Work out the finished part from the listing and answer in its coordinate system (mm). Round coordinates to 2 decimals unless told otherwise and drop trailing zeros. Order: outer loops, then holes, each group sorted by start corner. A loop starts at its lowest first (then second) coordinate and runs counter-clockwise, first axis right, second up. Notation, with made-up numbers: (-34.75, -4) - (-13.75, -4) arc R35 cw to (-13.75, 29) - close; hole circle Ø5 at (51, 85.5). An arc over 180 degrees is marked (long way). Use CSV: the item, a comma, the result in double quotes.
from build123d import *

# Parameters (mm, degrees)
CYLINDER107_R          = 1.8
CYLINDER107_DEPTH      = 34
CYLINDER107_ROLL_ANGLE = 90
CYLINDER106_R          = 1.8
CYLINDER106_DEPTH      = 34
CYLINDER106_ROLL_ANGLE = 90
CYLINDER109_R          = 1.8
CYLINDER109_DEPTH      = 34
CYLINDER109_ROLL_ANGLE = 90
CYLINDER108_R          = 1.8
CYLINDER108_DEPTH      = 34
CYLINDER108_ROLL_ANGLE = 90
BOX054_W               = 50
BOX054_H               = 6
BOX054_DEPTH           = 52


with BuildPart() as cilindro063:
    # Cylinder107 → Cylinder107 (new body)
    with BuildSketch(Plane.XY):
        Circle(CYLINDER107_R)
    extrude(amount=CYLINDER107_DEPTH)


with BuildPart() as cilindro063_1:
    # Cylinder107 roll: moved
    add(cilindro063.part.rotate(Axis((0, 0, 0), (1, 0, 0)), CYLINDER107_ROLL_ANGLE))


with BuildPart() as cilindro063_2:
    # Cylinder107 placement: moved
    add(cilindro063_1.part.moved(Location((16, -10, 63))))


with BuildPart() as fusion059:
    # Cylinder106 → Cylinder106 (new body)
    with BuildSketch(Plane.XY):
        Circle(CYLINDER106_R)
    extrude(amount=CYLINDER106_DEPTH)


with BuildPart() as fusion059_1:
    # Cylinder106 roll: moved
    add(fusion059.part.rotate(Axis((0, 0, 0), (1, 0, 0)), CYLINDER106_ROLL_ANGLE))


with BuildPart() as fusion059_2:
    # Cylinder106 placement: moved
    add(fusion059_1.part.moved(Location((50, -10, 63))))

    # Fusion059: union Cilindro063
    add(cilindro063_2.part)


with BuildPart() as cilindro065:
    # Cylinder109 → Cylinder109 (new body)
    with BuildSketch(Plane.XY):
        Circle(CYLINDER109_R)
    extrude(amount=CYLINDER109_DEPTH)


with BuildPart() as cilindro065_1:
    # Cylinder109 roll: moved
    add(cilindro065.part.rotate(Axis((0, 0, 0), (1, 0, 0)), CYLINDER109_ROLL_ANGLE))


with BuildPart() as cilindro065_2:
    # Cylinder109 placement: moved
    add(cilindro065_1.part.moved(Location((16, -10, 63))))


with BuildPart() as fusion061:
    # Cylinder108 → Cylinder108 (new body)
    with BuildSketch(Plane.XY):
        Circle(CYLINDER108_R)
    extrude(amount=CYLINDER108_DEPTH)


with BuildPart() as fusion061_1:
    # Cylinder108 roll: moved
    add(fusion061.part.rotate(Axis((0, 0, 0), (1, 0, 0)), CYLINDER108_ROLL_ANGLE))


with BuildPart() as fusion061_2:
    # Cylinder108 placement: moved
    add(fusion061_1.part.moved(Location((50, -10, 63))))

    # Fusion060: union Cilindro065
    add(cilindro065_2.part)


with BuildPart() as fusion061_3:
    # Fusion060 placement: moved
    add(fusion061_2.part.moved(Location((0, 0, 43))))

    # Fusion061: union Fusion059
    add(fusion059_2.part)


with BuildPart() as obj1:
    # Box054 → Box054 (new body)
    with BuildSketch(Plane(origin=(8, -23, 59), x_dir=(1, 0, 0), z_dir=(0, 0, 1))):
        with Locations((25, 3)):
            Rectangle(BOX054_W, BOX054_H)
    extrude(amount=BOX054_DEPTH)

    # Cut126: cut Fusion061
    add(fusion061_3.part, mode=Mode.SUBTRACT)


solid = obj1.part
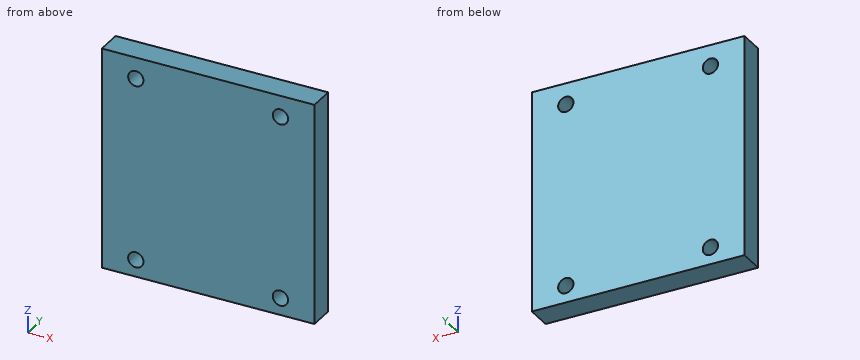
(1) Find section A-A (x = 50). Determine the outline of the cut face in (y, z), and give its area (3 significant figures).
Findings below:
outline,"(-23, 59) - (-17, 59) - (-17, 61.2) - (-23, 61.2) - close; (-23, 64.8) - (-17, 64.8) - (-17, 104.2) - (-23, 104.2) - close; (-23, 107.8) - (-17, 107.8) - (-17, 111) - (-23, 111) - close"
area,"269 mm²"
(2) Find section B-B (z = 106). Determine the outline of the cut face in (x, y).
Findings below:
outline,"(8, -23) - (14.2, -23) - (14.2, -17) - (8, -17) - close; (17.8, -23) - (48.2, -23) - (48.2, -17) - (17.8, -17) - close; (51.8, -23) - (58, -23) - (58, -17) - (51.8, -17) - close"
(3) Find the intervals of material crossed by L1, parallel to X at y = -20.9, z = 106; L2, parallel to Z at x = 50, y = -20.5; L3, parallel to X at y = -19, z = 107, in increasing order. Write a range as from..to.
Findings below:
L1,"x = 8..14.2, 17.8..48.2, 51.8..58"
L2,"z = 59..61.2, 64.8..104.2, 107.8..111"
L3,"x = 8..14.5, 17.5..48.5, 51.5..58"
(4) Find section C-C (y = -17.95). Determine the outline of the cut face in (x, z).
Findings below:
outline,"(8, 59) - (58, 59) - (58, 111) - (8, 111) - close; hole circle Ø3.6 at (16, 63); hole circle Ø3.6 at (16, 106); hole circle Ø3.6 at (50, 63); hole circle Ø3.6 at (50, 106)"
